Study the drawing (mm; zero at the part's minimum x, y, z) and answer. A direction names the side the tool comes from. Coordinates: 2 decimals unless noted, no trailing zeros. Write each loop counter-clockwise with the first axis right and the second up, starting at its lowest first coordinate (ties: lowest second). Pieces come first, ordered by that corner, then holes. Notation, with made-up numbers: (49.25, 3) - (92.25, 3) arc R10 ccw to (92.25, 15) - close; hole circle Ø10 at (80, 26.25). An arc over 180 degrees is marked (long way). One line per item, written item: value.
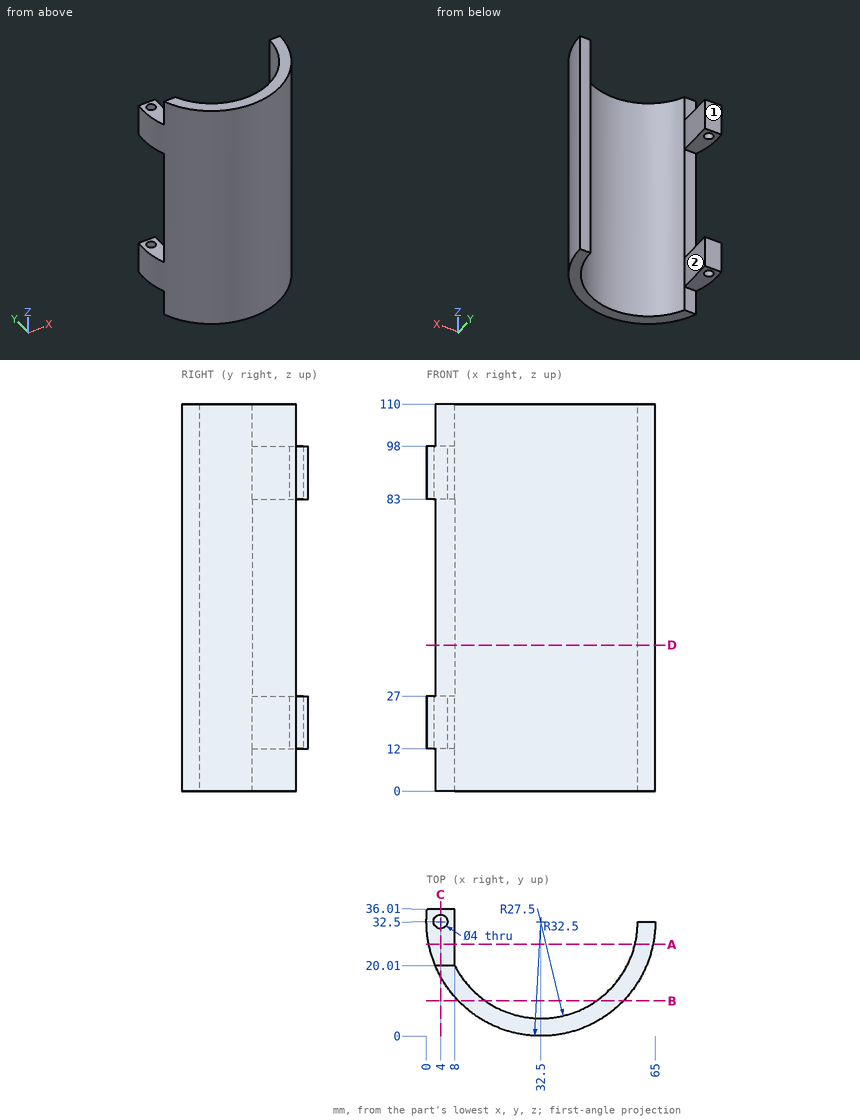
Item 1: Given pin 1 (4.5 mm diameter, centred on x = 4, y = 32.5, fed in from -Z); pin 2 (1.7 mm diameter, centred on x = 4, z = 6, fed in from +Y); pin 3 (2.5 mm diameter, centred on x = 4, y = 28.5, fed in from +Z), each flat-ended and moving along its own axis, determine where each tip first touches the part or whether it passes through.
Evaluation:
pin 1: stops at z = 12
pin 2: stops at y = 20.01
pin 3: stops at z = 98
Item 2: Section D-D, the plane z = 41.5 is taken. Determine the outline of the cut face in (x, y).
Evaluation:
outline: (2.5, 20.01) arc R32.5 ccw to (65, 32.5) - (60, 32.5) arc R27.5 cw to (8, 20.01) - close
Item 3: Consider probe 1 along X at (y, z) = (32, 91); probe 2 along X at (y, z) = (16.5, 36); probe 3 along Y at (x, z) = (4, 19.25). Determine where each line is inside the solid, lowest interval first.
Evaluation:
probe 1: x = 0 to 2.06, 5.94 to 8, 60 to 65
probe 2: x = 4.21 to 10.13, 54.87 to 60.79
probe 3: y = 16.88 to 30.5, 34.5 to 36.01
Item 4: Section A-A, the plane y = 26 is taken. Determine the outline of the cut face in (x, z), then the cut area to 3 significant figures.
Evaluation:
outline: (0.66, 12) - (8, 12) - (8, 27) - (0.66, 27) - close; (0.66, 83) - (8, 83) - (8, 98) - (0.66, 98) - close; (59.22, 0) - (64.34, 0) - (64.34, 110) - (59.22, 110) - close
area: 784 mm2
Item 5: Section B-B, the plane y = 10 is taken. Determine the outline of the cut face in (x, z), then the cut area to 3 significant figures.
Evaluation:
outline: (9.05, 0) - (16.69, 0) - (16.69, 110) - (9.05, 110) - close; (48.31, 0) - (55.95, 0) - (55.95, 110) - (48.31, 110) - close
area: 1,680 mm2
Item 6: Section C-C, the plane x = 4 is taken. Determine the outline of the cut face in (y, z), then the cut area to 3 significant figures.
Evaluation:
outline: (16.88, 0) - (20.01, 0) - (20.01, 12) - (30.5, 12) - (30.5, 27) - (20.01, 27) - (20.01, 83) - (30.5, 83) - (30.5, 98) - (20.01, 98) - (20.01, 110) - (16.88, 110) - close; (34.5, 12) - (36.01, 12) - (36.01, 27) - (34.5, 27) - close; (34.5, 83) - (36.01, 83) - (36.01, 98) - (34.5, 98) - close
area: 704 mm2
Item 7: Which of the six approach directions +Z, -Z, +X, -X, +Y, -Y give full straight-line access (tool end or side, diameter ignored) to the marked faces 1 and 2?
Evaluation:
face 1: +Z, -Z, +X, -X, +Y
face 2: +Z, -Z, +Y
